Model file for the job. Use its own axes, mm. Face numbers are marked on the shaded views. A direction names the side the tool comes from. Round coordinates to 2 decimals unless told otherwise and drop trailing zeros. Loops run counter-clockwise (first coordinate to the right, second up) from the corner with the lowest first, then second, coordinate; pieces in that order, holes last.
Autodesk Inventor part; units mm, degrees
ref_plane "РабПлоскость1" through (0, 0, 22) normal (0, 0, 1) x (1, 0, 0)
ref_plane "YZ Plane" through (0, 0, 0) normal (1, 0, 0) x (0, 1, 0)
ref_plane "XZ Plane" through (0, 0, 0) normal (0, 1, 0) x (-1, 0, 0)
sketch "Эскиз1" plane through (0, 0, 0) normal (0, 0, 1) x (1, 0, 0)
  line L0 (0, 0) -> (0, 4)
  line L1 (0, 4) -> (18, 4)
  line L2 (18, 4) -> (18, 11)
  line L3 (18, 11) -> (20, 11)
  line L4 (20, 11) -> (20, 18)
  line L5 (20, 18) -> (63.5, 18)
  line L6 (63.5, 18.25) -> (120.5, 18.25)
  line L7 (120.5, 18.25) -> (120.5, 18)
  line L8 (120.5, 18) -> (136.5, 18)
  line L9 (136.5, 18) -> (136.5, 0)
  line L10 (0, 0) -> (136.5, 0)
  line L11 (63.5, 18) -> (63.5, 18.25)
  point P0 (63, 17.5)
  point P1 (63, 17.5)
  dimension "d5" = 20
  dimension "d6" = 2
  dimension "d7" = 8
  dimension "d8" = 22
  dimension "d9" = 36
  dimension "d11" = 36.5
  dimension "d12" = 43.5
  dimension "d14" = 57
  dimension "d15" = 16
revolve "Вращение1" add sketch "Эскиз1" angle 360 about axis through (0, 0, 0) along (1, 0, 0)
fillet "Сопряжение1" radius 5 1 edges at (63.5, -18, 0)
sketch "Эскиз2" plane through (0, 0, 0) normal (0, 1, 0) x (-1, 0, 0)
  line L0 (0, 4) -> (0, -4)
  line L1 (0, -3.5) -> (-12, -3.5)
  line L2 (-12, -3.5) -> (-12, -6.5419)
  line L3 (-12, -6.5419) -> (0, -6.5419)
  line L4 (0, -3.1455) -> (0, -6.5419)
  point P0 (0, 0)
  point P1 (0, 0)
  dimension "d20" = 3.5
  dimension "d21" = 12
extrude "Выдавливание1" cut sketch "Эскиз2" along normal mid plane 10
ref_plane "РабПлоскость1" through (0, 0, 22) normal (0, 0, 1) x (1, 0, 0)
sketch "Эскиз3" plane through (0, 0, 22) normal (0, 0, 1) x (1, 0, 0)
  line L0 (110, 0) -> (110, -6)
  line L1 (118, -6) -> (118, 0)
  arc A0 (110, -6) -> (118, -6) centre (114, -6) ccw
  line L2 (110, 0) -> (118, 0) construction
  line L3 (110, 0) -> (110, 6)
  line L4 (118, 6) -> (118, 0)
  arc A1 (118, 6) -> (110, 6) centre (114, 6) ccw
  point P0 (0, 0)
  dimension "d23" = 12
  dimension "d24" = 8
  dimension "d25" = 110
extrude "Выдавливание2" cut sketch "Эскиз3" against normal blind 8
pattern_circular "Круговой массив1" count 4 over 360 about axis through (92, 0, 0) along (1, 0, 0) of "Выдавливание2"
sketch "Эскиз4" plane through (0, 0, 22) normal (0, 0, 1) x (1, 0, 0)
  line L0 (148, 9) -> (128.5, 9)
  line L1 (128.5, 9) -> (128.5, -9)
  line L2 (128.5, -9) -> (136.5, -9)
  line L3 (136.5, -18) -> (136.5, 18)
  point P0 (0, 0)
  point P1 (136.5, 9)
  dimension "d31" = 8
  dimension "d32" = 18
  dimension "d33" = 9
extrude "Выдавливание3" cut sketch "Эскиз4" against normal blind 12
sketch "Эскиз5" plane through (20, 0, 0) normal (-1, 0, 0) x (0, 0, 1)
  arc A0 (-3.5, -1.9365) -> (-3.5, 1.9365) centre (0, 0) ccw
  circle A1 centre (0, 0) radius 14
  line L0 (0, 0) -> (0, -31.2) construction
  line L1 (0, 0) -> (9.8995, -9.8995) construction
  point P0 (9.8995, 9.8995)
  point P1 (-9.8995, 9.8995)
  point P2 (-9.8995, -9.8995)
  dimension "d43" = 28
  dimension "d44" = 45
  dimension "d47" = 360
hole "Отверстие1" at (20, -9.8995, 9.8995) at (20, 9.8995, 9.8995) at (20, 9.8995, -9.8995) at (20, -9.8995, -9.8995) direction (1, 0, 0) diameter 3.242 depth 5.2 tip angle 118
properties part number "CHP-42GP-775 ABHL" material "Алюминий 6061-AHC"
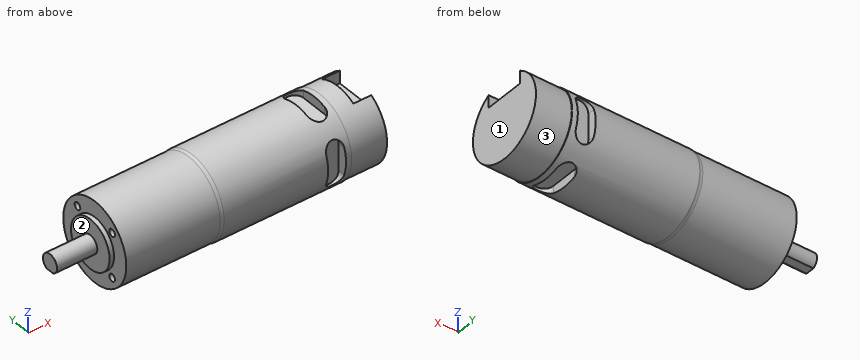
Q1. Tool access for the marked faces 1, 2 and 3: list every direction of +Z, -Z, +X, -X, +Y, -Y with a clear straight run to the whole face (end or side of a thin tool).
Q2. Slice it at B-B on z = 0. Give the cut face in (x, y).
Q3. Probe line 1 (X direction, y = 8, z = -4.5); line 2 (X direction, y = 8, z = -16); line 3 (X direction, y = 11.5, z = -13). List the from-to ranges inside material, lowest first.
Q4. Flat gauge pins, fed straight in: P1, Ø4, axis at x = 112.5, z = 0.5, coming from the +Y side; P2, Ø3, axis at x = 100.5, y = 3, coming from the +Z side; P3, Ø4, axis at x = 117, y = 10.5, coming from the -Z side. Where does each tip first touch, or does it go through?
Q5. Slice it at C-C on x = 91.5. Give the cut face in (y, z), plus the area to 3 significant figures.
Reply:
1. face 1: +Z, -Z, +X, +Y, -Y
1. face 2: -X
1. face 3: +X
2. outline: (0, -4) - (18, -4) - (18, -11) - (20, -11) - (20, -18) - (61.94, -18) arc R5 cw to (63.5, -18.25) - (110, -18.25) - (110, -14) - (118, -14) - (118, -18.25) - (120.5, -18.25) - (120.5, -18) - (136.5, -18) - (136.5, 18) - (120.5, 18) - (120.5, 18.25) - (118, 18.25) - (118, 14) - (110, 14) - (110, 18.25) - (63.5, 18.25) arc R5 cw to (61.94, 18) - (20, 18) - (20, 11) - (18, 11) - (18, 4) - (0, 4) - close
3. line 1: x = 18 to 136.5
3. line 2: x = 20 to 110.54, 117.46 to 136.5
3. line 3: x = 20 to 136.5
4. P1: stops at y = 14
4. P2: stops at z = 18.19
4. P3: stops at z = -16.15
5. outline: circle Ø36.5 at (0, 0)
5. area: 1,050 mm2
